The drawing under review shows one solid part. Ordinate dimensions are in mm from its lowest x, y, z. A direction names the side the tool comes from. Round coordinates to 2 decimals unless told otherwise and drop trailing zeros. Order: outer loops, then holes, each group sorted by start corner. A loop starts at its lowest first (then second) coordinate and runs counter-clockwise, first axis right, second up.
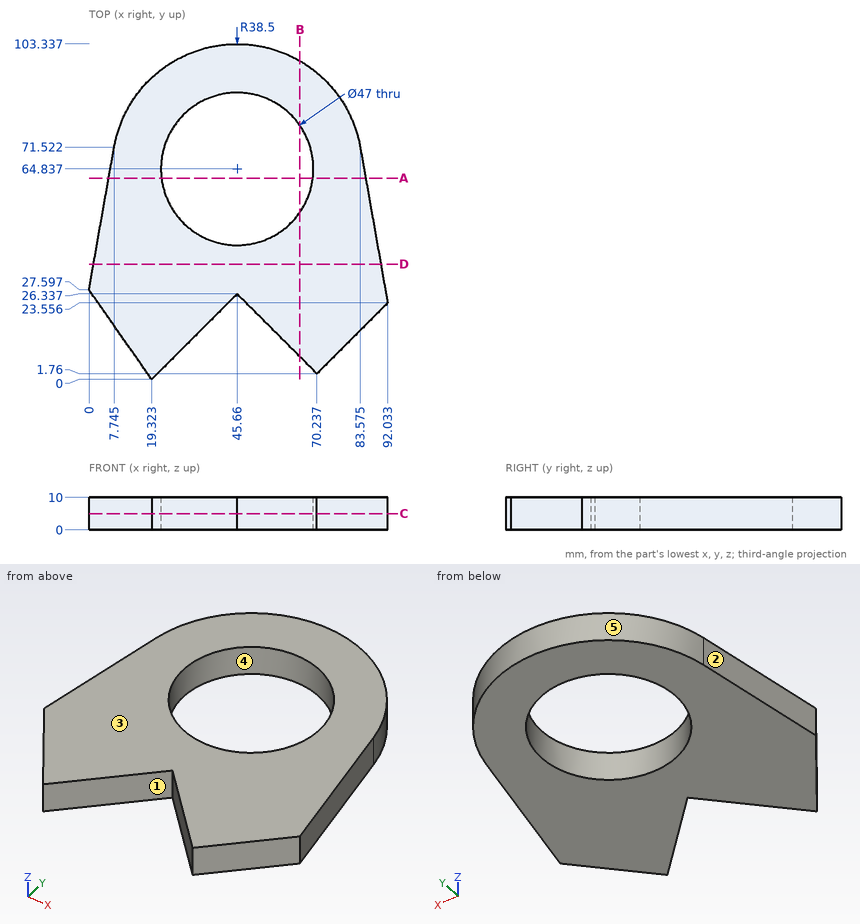
Q1. Clearance check with flat-ended pins moving along their axes: pin 1 (2 mm diameter, centred on x = 78.5, z = 1.5, fed in from +Y); pin 2 (3 mm diameter, centred on y = 64, z = 3.5, fed in from -X) (1 decimal); pin 3 (4 mm diameter, centred on x = 60.5, z = 6, fed in from +Y). State where each tip first meets the part, or that it passes through.
Q2. Wall thickness on line 1 (X direction, y = 4, z = 6.25) (1 decimal); line 2 (X direction, y = 44.5, z = 7) (1 decimal); line 3 (Y direction, x = 30.5, z = 5.5) (1 decimal): over which ranges is each line inside the solid? List them lowest first.
Q3. Take a section at A-A, the plane y = 62. State the section outline as (x, z) points (1 decimal).
Q4. Take a section at D-D, the plane y = 35.5. State the section outline as (x, z) points.
Q5. Tool access review of the marked faces 1 and 2: name each direction out of +Z, -Z, +X, -X, +Y, -Y from which nothing blocks a thin tool from reaching the whole face with its end or side.
Q6. Take a section at B-B, the plane x = 65. State the section outline as (y, z) points, plus the area to 3 significant figures.
Q7. Take a section at C-C, the plane z = 5. State the section outline as (x, y) points (1 decimal).
Q8. Mouldability with a two-part tool opening along Y and no side actions: class the marked faces 3, 4 and 5 as +Y half, -Y half, draft (parallel to the pull), parting line (faces both ways), or undercut.
Working result:
1. pin 1: stops at y = 86.48
1. pin 2: stops at x = 6.2
1. pin 3: stops at y = 101.13
2. line 1: x = 16.5 to 23.3, 68 to 72.5
2. line 2: x = 3 to 33.9, 57.4 to 88.3
2. line 3: y = 11.2 to 46.9, 82.8 to 100.2
3. outline: (6.1, 0) - (22.3, 0) - (22.3, 10) - (6.1, 10) - close; (69, 0) - (85.3, 0) - (85.3, 10) - (69, 10) - close
4. outline: (1.39, 0) - (89.93, 0) - (89.93, 10) - (1.39, 10) - close
5. face 1: +Z, -Z, -Y
5. face 2: +Z, -Z, -X, +Y
6. outline: (7, 0) - (51.49, 0) - (51.49, 10) - (7, 10) - close; (78.19, 0) - (98.13, 0) - (98.13, 10) - (78.19, 10) - close
6. area: 644 mm2
7. outline: (0, 27.6) - (19.3, 0) - (45.7, 26.3) - (70.2, 1.8) - (92, 23.6) - (83.6, 71.5) arc R38.5 ccw to (7.7, 71.5) - close; hole circle Ø47 at (45.7, 64.8)
8. face 3: draft
8. face 4: undercut
8. face 5: +Y half
